Here's how the part is built. I have some questions about the finished solid (model axes, mm). A direction names the side the tool comes from. Coordinates: 2 decimals unless noted, no trailing zeros. Loops run counter-clockwise (first coordinate to the right, second up) from the corner with the lowest first, then second, coordinate; pieces in that order, holes last. Notation, with made-up numbers: M 35.25,49.5 L 61.25,49.5 A22 ccw 61.25,55.5 Z; hole C -27.5,57 d6. An arc over 180 degrees is marked long. Use CSV: the item, a comma, the result in double quotes. Start each with the question number.
Q1. If we section it at A-A (x = 0): Please give me the cut outline in (y, z).
Q2. If we mould it in two halves opening along Y, with no side actions, what happens to faces 3 (the cylindrical face through (4.455, 20.061, 5.316)), 4 (the conical face through (4.24, 19.08, 11.78)), 5 (the flat face through (-18, 7, 0))? For each: +Y half, -Y half, draft (parallel to the pull), parting line (faces both ways), or undercut.
Q3. If we section it at C-C (z = 23): Please give me the cut outline in (x, y), and give its area (3 significant figures).
Q4. If we section it at D-D (z = 17): Please give me the cut outline in (x, y).
Q5. Please list where these lines run through material, in increasing order: probe 1 along X at (y, z) = (-13, 20); probe 2 along X at (y, z) = (13, 9); probe 3 along Y at (x, z) = (10.5, 4) (3 decimals). Write a range as [from, to].
Q6. For pin 1 Ø3 at (x, z) = (12.5, 31.5) entering from +Y; pin 2 Ø1 at (x, z) = (-7.5, 21) entering from +Y; pin 3 Ø5 at (y, z) = (12, 25.5) entering from -X, each with a flat end and sliding along its axis, tell me the tip position at first contact or that it passes through.
Q7. Which directions (+Z, -Z, +X, -X, +Y, -Y) give clear straight access to the entire face, cutting with the end or side of a thin tool? Please do faces 1 (the conical face through (4.66, 20.99, 20.49)), 2 (the cylindrical face through (-20.03, 6.31, 32.7)).
Autodesk Inventor part; units mm, degrees
ref_plane "YZ Plane" through (0, 0, 0) normal (1, 0, 0) x (0, 1, 0)
ref_plane "XZ Plane" through (0, 0, 0) normal (0, 1, 0) x (-1, 0, 0)
ref_plane "XY Plane" through (0, 0, 0) normal (0, 0, 1) x (1, 0, 0)
sketch "Sketch1" plane through (0, 0, 0) normal (0, 1, 0) x (-1, 0, 0)
  line L0 (0, 0) -> (0, 37)
  line L1 (20.55, 0) -> (20.55, 10)
  line L2 (20.55, 10) -> (23, 37)
  line L3 (23, 37) -> (21, 37)
  line L4 (18.55, 0) -> (20.55, 0)
  line L5 (0, 0) -> (18.55, 0) construction
  line L6 (21, 37) -> (0, 37) construction
  line L7 (21, 37) -> (21, 29)
  line L8 (21, 29) -> (18.55, 0)
  dimension "d0" = 41.1
  dimension "d1" = 42
  dimension "d2" = 37
  dimension "d3" = 10
  dimension "d4" = 8
  dimension "d11" = 2
  dimension "d12" = 2
revolve "Revolution1" add sketch "Sketch1" angle 360 about axis through (0, 0, 0) along (0, 0, 1)
chamfer "Chamfer1" distance 0.5 angle 45 4 edges at (20.55, 0, 0) (18.55, 0, 0) (23, 0, 37) (21, 0, 37)
properties part number "Takumar-to-RisingCam" material "ABS Plastic"
Results below:
1,outline,"M -22.95,36.5 L -20.55,10 L -20.55,0.5 L -20.05,0 L -19.05,0 L -18.59,0.5 L -21,29 L -21,36.5 L -21.5,37 L -22.5,37 Z; M 18.59,0.5 L 19.05,0 L 20.05,0 L 20.55,0.5 L 20.55,10 L 22.95,36.5 L 22.5,37 L 21.5,37 L 21,36.5 L 21,29 Z"
2,face 3,"parting line"
2,face 4,"undercut"
2,face 5,"draft"
3,outline,"C 0,0 d43.46; hole C 0,0 d40.99"
3,area,"164 mm^2"
4,outline,"C 0,0 d42.37; hole C 0,0 d39.97"
5,probe 1,"[-17.07, -15.51], [15.51, 17.07]"
5,probe 2,"[-15.92, -14.28], [14.28, 15.92]"
5,probe 3,"[-17.665, -15.7], [15.7, 17.665]"
6,pin 1,"y = 19.64"
6,pin 2,"y = 20.39"
6,pin 3,"x = -19.82"
7,face 1,"-Z"
7,face 2,"+Z"
